```python
from build123d import *

# Parameters (mm, degrees)
F0_W     = 50
F0_H     = 50
F1_DEPTH = 30
F2_W     = 50
F2_H     = 30
F2_H_2   = 55
F3_DEPTH = 3.175
F4_R     = 5


# Not quite as in the source:
# - an extrude whose draft closes it to a point is written as a loft to that point


with BuildPart() as f1:
    # F0 (on Top) → F1 (new body)
    with BuildSketch(Plane.XY):
        with Locations((-20.7551017412, -14.590555802)):
            Rectangle(F0_W, F0_H)
    extrude(amount=F1_DEPTH)

    # F2 (on face) → F3 (join)
    with BuildSketch(Plane(origin=(0, 10.409444198, 0), x_dir=(-1, 0, 0), z_dir=(0, 1, 0))):
        with Locations((20.7551017412, 15)):
            Rectangle(F2_W, F2_H)
        with Locations((20.7551017412, 57.5)):
            Rectangle(F2_W, F2_H_2)
    extrude(amount=F3_DEPTH)

    # F4 (on face) → F5 section 0
    with BuildSketch(Plane(origin=(0, 0, 0), x_dir=(1, 0, 0), z_dir=(0, 0, -1)), mode=Mode.PRIVATE) as f5_s0:
        with Locations((-20.7551017412, 14.5431621725)):
            Circle(F4_R)
    loft([f5_s0.sketch, Vertex(-20.7551017412, -14.5431621725, -5.958767963)], ruled=True)


solid = f1.part
```
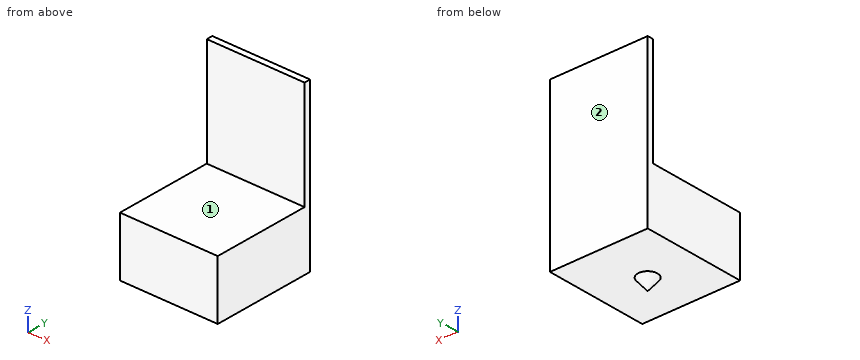
Verification items for the finished model (mm, model axes). Face numbers are marked on the shaded views. A direction names the side the tool comes from. Coordinates: 2 decimals unless noted, no trailing zeros. Write each loop counter-clockwise with the first axis right and the second up, starting at its lowest first coordinate (ties: lowest second). Pieces come first, ordered by that corner, then holes. Notation, with made-up numbers: (60.25, -11.75) - (95.25, -11.75) arc R22 cw to (95.25, 8.25) - close; hole circle Ø9 at (31.25, 80.5). An arc over 180 degrees is marked (long way). One line per question, with ' | ' between items. Start each with the question number.
1. Section check C-C (z = 49). Enter the section's corners in (x, y), plus the area to 3 significant figures.
2. Access from +Z, -Z, +X, -X, +Y, -Y to the whole of each face (thin tool, end or side, straight path). Record for the marked faces 1 and 2.
3. Material ranges on line 1 along Z through (x, y) = (-19, -9.5); line 2 along Y through (x, z) = (-9.5, 35); line 3 along Z through (x, y) = (-7.5, 10.5), recorded low to high.
4. Gauge pin test, flat ends, axial feed: P1, Ø6, axis at x = -15.5, y = -13.5, coming from the +Z side; P2, Ø25, axis at x = -27, z = 63, coming from the -Y side; P3, Ø15, axis at x = -16, y = -13.5, coming from the -Z side. Record the tip position at first contact, or that the pin passes through.
5. Section check A-A (x = -3.5). Enter the section's corners in (y, z).
6. Section check B-B (y = -24). Enter the section's corners in (x, z), plus the area to 3 significant figures.
Computed values:
1) outline: (-45.76, 10.41) - (4.24, 10.41) - (4.24, 13.58) - (-45.76, 13.58) - close | area: 159 mm²
2) face 1: +Z, +X, -X, -Y | face 2: +Z, -Z, +X, -X, +Y
3) line 1: 0 to 30 | line 2: 10.41 to 13.58 | line 3: 0 to 85
4) P1: z = 30 | P2: y = 10.41 | P3: z = -5.96
5) outline: (-39.59, 0) - (13.58, 0) - (13.58, 85) - (10.41, 85) - (10.41, 30) - (-39.59, 30) - close
6) outline: (-45.76, 0) - (4.24, 0) - (4.24, 30) - (-45.76, 30) - close | area: 1,500 mm²
